Verification items for the finished model (mm, model axes). A direction names the side the tool comes from. Round coordinates to 2 decimals unless told otherwise and drop trailing zeros. Write each loop counter-clockwise with the first axis right and the second up, starting at its lowest first coordinate (ties: lowest second). Pieces come first, ordered by that corner, then holes. Notation, with made-up numbers: M 62.5,-1.5 L 116.5,-1.5 A21 cw 116.5,29.5 Z; hole C -31.5,87 d5. An arc over 180 degrees is marked long. One line per question, with ' | ' between items. Start each with the question number.
Q1. Cross-section at B-B (x = 24). Record the boundary of the cut face in (y, z).
Q2. Release check for a two-part mould opening along Z. For faces 6 (the face through (26, 29, 3.2)), 7 (the face through (27, 28, -8)), 8 (the face through (0, 19, 10)), 9 (the face through (-26, 29, -6.8)) record: released by +Z, released by -Z, zero draft, split by the parting line, or undercut.
Q3. Thickness scan on line 1 along Z through (x, y) = (-24, 28.2); line 2 along X through (y, z) = (17, -9); line 3 along Y through (x, z) = (-18.5, -1.5). Record the ranges inside material, lowest first. Write a range as from..to.
Q4. Cross-section at C-C (z = 8.5). Record the boundary of the cut face in (x, y), then the cut area to 3 significant figures.
Q5. Gauge pin test, flat ends, axial feed: pin 1 (2.5 mm diameter, centred on y = 29, z = 9, fed in from +X); pin 2 (6.5 mm diameter, centred on x = -24, z = 5, fed in from +Y); pin 3 (1.5 mm diameter, centred on x = -21, z = -5.5, fed in from +Y). Record the tip position at first contact, or that the pin passes through.
Q6. Cross-section at A-A (x = -24). Record the boundary of the cut face in (y, z).
Q7. Cross-section at D-D (x = 11). Record the boundary of the cut face in (y, z).
Q8. Tool access check on faces 1 (the face through (25, 3.333, 0)), 2 (the face through (26, 29, -3.2)), 3 (the face through (-26, 29, -3.2)), 4 (the face through (-20.5, 13, 0)), 5 (the face through (24, 30, 0)). Record the directions out of +Z, -Z, +X, -X, +Y, -Y that give a thin tool (end or side, any length) a straight path to the whole face; none if there is none.
from build123d import *

# Parameters (mm, degrees)
SKETCH_1_W          = 41
SKETCH_1_H          = 20
EXTRUDE_1_DEPTH     = 38
SKETCH_2_W          = 54
SKETCH_2_H          = 20
EXTRUDE_2_DEPTH     = 3
CUT_EXTRUDE_1_REACH = 43.581
SKETCH_4_R          = 7.5
EXTRUDE_3_DEPTH     = 3
SKETCH_5_R          = 3
EXTRUDE_4_DEPTH     = 5.5
SKETCH_6_W          = 7.726872992
SKETCH_6_H          = 2.816336885
EXTRUDE_5_DEPTH     = 10


with BuildPart() as part:
    # 草圖1 → 伸長1 (new body)
    with BuildSketch(Plane(origin=(0, 0, 0), x_dir=(1, 0, 0), z_dir=(0, 1, 0))):
        Rectangle(SKETCH_1_W, SKETCH_1_H)
    extrude(amount=EXTRUDE_1_DEPTH)

    # 草圖2 → 伸長2 (add)
    with BuildSketch(Plane(origin=(0, 27, 0), x_dir=(-1, 0, 0), z_dir=(0, 1, 0))):
        Rectangle(SKETCH_2_W, SKETCH_2_H)
    extrude(amount=EXTRUDE_2_DEPTH)

    # 草圖3 → 除料-伸長1 (cut, up to next)
    with BuildSketch(Plane(origin=(0, 30, 0), x_dir=(-1, 0, 0), z_dir=(0, 1, 0)), mode=Mode.PRIVATE) as cut_extrude_1_sk1:
        with BuildLine():
            Line((-27, 3.2), (-24.871779789, 3.2))
            ThreePointArc((-24.871779789, 3.2), (-22, 5), (-24.871779789, 6.8))
            Line((-24.871779789, 6.8), (-27, 6.8))
            Line((-27, 6.8), (-27, 3.2))
        make_face()
    cut_extrude_1_tool1 = extrude(cut_extrude_1_sk1.sketch, amount=-CUT_EXTRUDE_1_REACH, mode=Mode.PRIVATE) & part.part
    # 草圖3 → 除料-伸長1 (cut, up to next)
    with BuildSketch(Plane(origin=(0, 30, 0), x_dir=(-1, 0, 0), z_dir=(0, 1, 0)), mode=Mode.PRIVATE) as cut_extrude_1_sk2:
        with BuildLine():
            Line((-27, -6.8), (-24.871779789, -6.8))
            ThreePointArc((-24.871779789, -6.8), (-22, -5), (-24.871779789, -3.2))
            Line((-24.871779789, -3.2), (-27, -3.2))
            Line((-27, -3.2), (-27, -6.8))
        make_face()
    cut_extrude_1_tool2 = extrude(cut_extrude_1_sk2.sketch, amount=-CUT_EXTRUDE_1_REACH, mode=Mode.PRIVATE) & part.part
    # 草圖3 → 除料-伸長1 (cut, up to next)
    with BuildSketch(Plane(origin=(0, 30, 0), x_dir=(-1, 0, 0), z_dir=(0, 1, 0)), mode=Mode.PRIVATE) as cut_extrude_1_sk3:
        with BuildLine():
            Line((27, -3.2), (24.871779789, -3.2))
            ThreePointArc((24.871779789, -3.2), (22, -5), (24.871779789, -6.8))
            Line((24.871779789, -6.8), (27, -6.8))
            Line((27, -6.8), (27, -3.2))
        make_face()
    cut_extrude_1_tool3 = extrude(cut_extrude_1_sk3.sketch, amount=-CUT_EXTRUDE_1_REACH, mode=Mode.PRIVATE) & part.part
    # 草圖3 → 除料-伸長1 (cut, up to next)
    with BuildSketch(Plane(origin=(0, 30, 0), x_dir=(-1, 0, 0), z_dir=(0, 1, 0)), mode=Mode.PRIVATE) as cut_extrude_1_sk4:
        with BuildLine():
            Line((27, 6.8), (24.871779789, 6.8))
            ThreePointArc((24.871779789, 6.8), (22, 5), (24.871779789, 3.2))
            Line((24.871779789, 3.2), (27, 3.2))
            Line((27, 3.2), (27, 6.8))
        make_face()
    cut_extrude_1_tool4 = extrude(cut_extrude_1_sk4.sketch, amount=-CUT_EXTRUDE_1_REACH, mode=Mode.PRIVATE) & part.part
    add(cut_extrude_1_tool1.solids().sort_by_distance((24.63194, 30, 5))[0], mode=Mode.SUBTRACT)
    add(cut_extrude_1_tool2.solids().sort_by_distance((24.63194, 30, -5))[0], mode=Mode.SUBTRACT)
    add(cut_extrude_1_tool3.solids().sort_by_distance((-24.63194, 30, -5))[0], mode=Mode.SUBTRACT)
    add(cut_extrude_1_tool4.solids().sort_by_distance((-24.63194, 30, 5))[0], mode=Mode.SUBTRACT)

    # 草圖4 → 伸長3 (add)
    with BuildSketch(Plane(origin=(0, 30, 0), x_dir=(-1, 0, 0), z_dir=(0, 1, 0))):
        with Locations((-11, 0)):
            Circle(SKETCH_4_R)
    extrude(amount=EXTRUDE_3_DEPTH)

    # 草圖5 → 伸長4 (add)
    with BuildSketch(Plane(origin=(0, 38, 0), x_dir=(-1, 0, 0), z_dir=(0, 1, 0))):
        with Locations(Location((-11, 0, 0), (0, 0, 90))):
            Circle(SKETCH_5_R)
    extrude(amount=EXTRUDE_4_DEPTH)

    # 草圖6 → 伸長5 (add)
    with BuildSketch(Plane(origin=(20.5, 0, 0), x_dir=(0, 0, -1), z_dir=(1, 0, 0))):
        with Locations((0.541603247, 4.740833757)):
            Rectangle(SKETCH_6_W, SKETCH_6_H)
    extrude(amount=EXTRUDE_5_DEPTH)


solid = part.part
Determined:
1) outline: M 3.33,-4.41 L 6.15,-4.41 L 6.15,3.32 L 3.33,3.32 Z; M 27,-10 L 30,-10 L 30,-7 L 27,-7 Z; M 27,-3 L 30,-3 L 30,3 L 27,3 Z; M 27,7 L 30,7 L 30,10 L 27,10 Z
2) face 6: undercut | face 7: zero draft | face 8: released by +Z | face 9: undercut
3) line 1: z = -10..-7, -3..3, 7..10 | line 2: x = -20.5..20.5 | line 3: y = 0..38
4) outline: M -27,27 L -20.5,27 L -20.5,0 L 20.5,0 L 20.5,27 L 27,27 L 27,30 L 20.5,30 L 20.5,38 L -20.5,38 L -20.5,30 L -27,30 Z | area: 1,600 mm²
5) pin 1: stops at x = 27 | pin 2: stops at y = 30 | pin 3: stops at y = 38
6) outline: M 27,-10 L 30,-10 L 30,-7 L 27,-7 Z; M 27,-3 L 30,-3 L 30,3 L 27,3 Z; M 27,7 L 30,7 L 30,10 L 27,10 Z
7) outline: M 0,-10 L 38,-10 L 38,-3 L 43.5,-3 L 43.5,3 L 38,3 L 38,10 L 0,10 Z
8) face 1: +Z, -Z, +X, -Y | face 2: +X, +Y | face 3: -X, +Y, -Y | face 4: +Z, -Z, -X, -Y | face 5: +Z, -Z, +X, +Y
